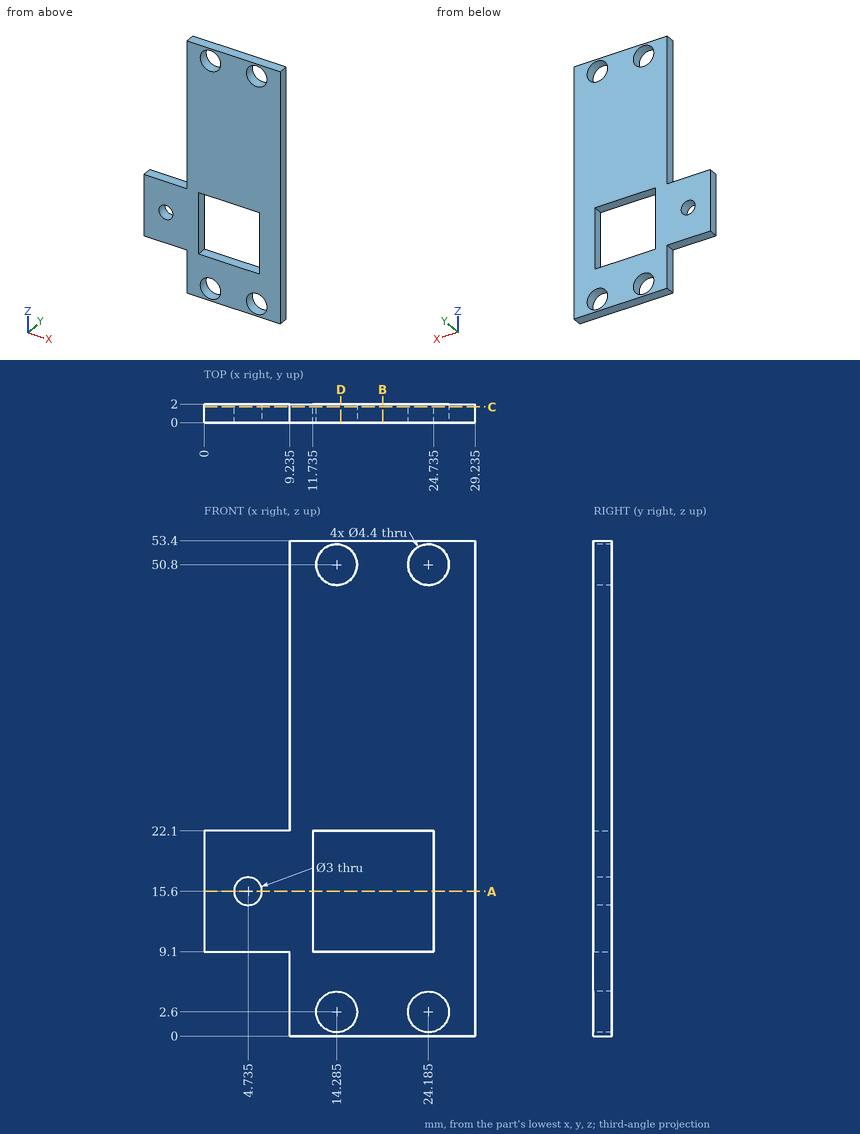
Design review of the part shown in the three views and the two pictorial views. Dimensions are in mm from the part's minimum x, y and z. Coordinates: 2 decimals unless noted, no trailing zeros. Write each loop counter-clockwise with the first axis right and the second up, starting at its lowest first coordinate (ties: lowest second). Pieces come first, ordered by that corner, then holes.
1) We need section A-A on z = 15.6. State the section outline as (x, y) points (3 decimals).
2) We need section C-C on y = 1.7. State the section outline as (x, z) points (3 decimals).
3) We need section D-D on x = 14.75. State the section outline as (y, z) points, then the cut area to 3 significant figures.
4) To check wall thickness, follow probe 1 along Z at (x, y) = (4.75, 1); probe 2 along Z at (x, y) = (21.5, 1.4); probe 3 along Z at (x, y) = (13.75, 1.6). State the ranges of each line that lie inside material, in increasing order.
5) We need section B-B on x = 19.25. State the section outline as (y, z) points.
6) Clearance check with flat-ended pins moving along their axes: pin 1 Ø0.6 at (y, z) = (1, 5.5) entering from -X (3 decimals); pin 2 Ø0.6 at (x, y) = (4.5, 1.5) entering from +Z; pin 3 Ø1 at (x, y) = (2.5, 1) entering from -Z. State where each tip first meets the part, or that it passes through.
Answer list:
1. outline: (0, 0) - (3.235, 0) - (3.235, 2) - (0, 2) - close; (6.235, 0) - (11.735, 0) - (11.735, 2) - (6.235, 2) - close; (24.735, 0) - (29.235, 0) - (29.235, 2) - (24.735, 2) - close
2. outline: (0, 9.1) - (9.235, 9.1) - (9.235, 0) - (29.235, 0) - (29.235, 53.4) - (9.235, 53.4) - (9.235, 22.1) - (0, 22.1) - close; hole circle Ø3 at (4.735, 15.6); hole (11.735, 9.1) - (24.735, 9.1) - (24.735, 22.1) - (11.735, 22.1) - close; hole circle Ø4.4 at (14.285, 2.6); hole circle Ø4.4 at (14.285, 50.8); hole circle Ø4.4 at (24.185, 2.6); hole circle Ø4.4 at (24.185, 50.8)
3. outline: (0, 0) - (2, 0) - (2, 0.45) - (0, 0.45) - close; (0, 4.75) - (2, 4.75) - (2, 9.1) - (0, 9.1) - close; (0, 22.1) - (2, 22.1) - (2, 48.65) - (0, 48.65) - close; (0, 52.95) - (2, 52.95) - (2, 53.4) - (0, 53.4) - close
3. area: 63.6 mm2
4. probe 1: z = 9.1 to 14.1, 17.1 to 22.1
4. probe 2: z = 0 to 9.1, 22.1 to 53.4
4. probe 3: z = 0 to 0.47, 4.73 to 9.1, 22.1 to 48.67, 52.93 to 53.4
5. outline: (0, 0) - (2, 0) - (2, 9.1) - (0, 9.1) - close; (0, 22.1) - (2, 22.1) - (2, 53.4) - (0, 53.4) - close
6. pin 1: stops at x = 9.235
6. pin 2: stops at z = 22.1
6. pin 3: stops at z = 9.1
